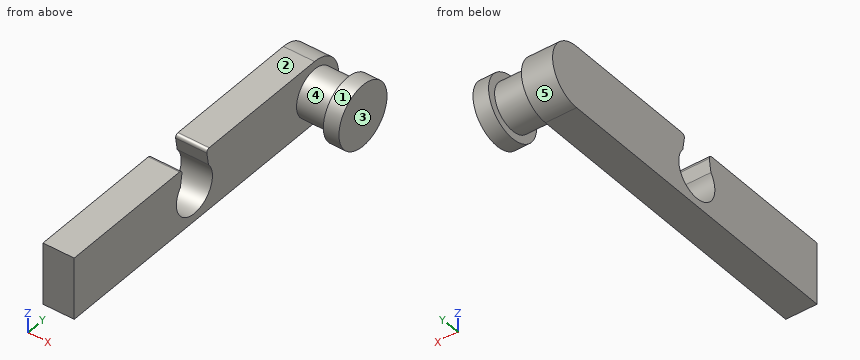
from build123d import *

# Parameters (mm, degrees)
BASE_DEPTH         = 2
ESQUISSE2_R        = 1.5
BOSS_FIX_DEPTH     = 2.1
ESQUISSE3_R        = 2
BOSS_BLOCAGE_DEPTH = 1
VIDE_TIGE_DEPTH    = 2
CONGE_TIGE_R       = 0.2


with BuildPart() as part:
    # Esquisse1 → BASE (new body)
    with BuildSketch(Plane(origin=(0, 0, 0), x_dir=(0, 0, -1), z_dir=(1, 0, 0))):
        with BuildLine():
            Line((2, 10), (2, -10))
            Line((2, -10), (-2, -10))
            Line((-2, -10), (-2, 10))
            ThreePointArc((-2, 10), (0, 12), (2, 10))
        make_face()
    extrude(amount=BASE_DEPTH)

    # Esquisse2 → BOSS FIX (add)
    with BuildSketch(Plane(origin=(2, 0, 0), x_dir=(0, 0, -1), z_dir=(1, 0, 0))):
        with Locations((0, 10)):
            Circle(ESQUISSE2_R)
    extrude(amount=BOSS_FIX_DEPTH)

    # Esquisse3 → BOSS BLOCAGE (add)
    with BuildSketch(Plane(origin=(4.1, 0, 0), x_dir=(0, 0, -1), z_dir=(1, 0, 0))):
        with Locations((0, 10)):
            Circle(ESQUISSE3_R)
    extrude(amount=BOSS_BLOCAGE_DEPTH)

    # Esquisse4 → VIDE TIGE (cut)
    with BuildSketch(Plane.ZY):
        with BuildLine():
            Line((2, 1), (0.937042571, 1.171303214))
            ThreePointArc((0.937042571, 1.171303214), (-1.5, 0), (0.937042571, -1.171303214))
            Line((0.937042571, -1.171303214), (2, -1))
            Line((2, -1), (2, 1))
        make_face()
    extrude(amount=-VIDE_TIGE_DEPTH, mode=Mode.SUBTRACT)

    # CONGE TIGE
    conge_tige_edges = [part.edges().sort_by_distance(p)[0] for p in [
        (1, -1, 2),
        (1, 1, 2),
    ]]
    fillet(conge_tige_edges, radius=CONGE_TIGE_R)


solid = part.part
Model file for the job. Use its own axes, mm. Face numbers are marked on the shaded views. A direction names the side the tool comes from. Coordinates: 2 decimals unless noted, no trailing zeros. Order: outer loops, then holes, each group sorted by start corner. A loop starts at its lowest first (then second) coordinate and runs counter-clockwise, first axis right, second up. Notation, with made-up numbers: (20, 60.5) -> (45, 60.5) arc R12 cw to (45, 67.5) -> close; hole circle Ø2 at (40.5, -33.75). An arc over 180 degrees is marked (long way). Return JSON: item names as keys, results as strings. Group by question number.
Item 1: Saw through at A-A on z = 0. Write the cut outline in (x, y), then the cut area to 3 significant figures.
Item 2: Pull direction X, two halves, no side cores. Call the marked faces 3, 4 and 5: pulls with the +X half, pulls with the -X half, needs draft (parallel to the pull), parting line crosses it, or undercut.
Item 3: Wall check: line 1 along Y through (x, z) = (0.45, 0); line 2 along X through (y, z) = (-5.5, 1.85); line 3 along Z through (x, y) = (1.15, 0). Give the ranges that are in metal, low to high. Write a range as [from, to].
Item 4: Saw through at B-B on x = 4.5. Write the cut outline in (y, z).
Item 5: Saw through at D-D on x = 2.6. Write the cut outline in (y, z).
Item 6: Tool access for the marked faces 1 and 2: list every direction of +Z, -Z, +X, -X, +Y, -Y with a clear straight run to the whole face (end or side of a thin tool).
Item 7: Saw through at C-C on y = 0. Write the cut outline in (x, z).
Values found:
{
 "1": {"outline": "(0, -10) -> (2, -10) -> (2, -1.5) -> (0, -1.5) -> close; (0, 1.5) -> (2, 1.5) -> (2, 8.5) -> (4.1, 8.5) -> (4.1, 8) -> (5.1, 8) -> (5.1, 12) -> (4.1, 12) -> (4.1, 11.5) -> (2, 11.5) -> (2, 12) -> (0, 12) -> close", "area": "48.3 mm2"},
 "2": {"face 3": "pulls with the +X half", "face 4": "undercut", "face 5": "needs draft"},
 "3": {"line 1": "y = [-10, -1.5], [1.5, 12]", "line 2": "x = [0, 2]", "line 3": "z = [-2, -1.5]"},
 "4": {"outline": "circle Ø4 at (10, 0)"},
 "5": {"outline": "circle Ø3 at (10, 0)"},
 "6": {"face 1": "+X", "face 2": "+Z, +X, -X, +Y, -Y"},
 "7": {"outline": "(0, -2) -> (2, -2) -> (2, -1.5) -> (0, -1.5) -> close"}
}
